Verification items for the finished model (mm, model axes). Face numbers are marked on the shaded views. Round coordinates to 2 decimals unless told otherwise and drop trailing zeros. Order: outer loops, then holes, each group sorted by start corner. A loop starts at its lowest first (then second) coordinate and runs counter-clockwise, first axis right, second up. Notation, with made-up numbers: (59.25, -26) -> (80.25, -26) arc R16 ccw to (80.25, -20) -> close; hole circle Ø6 at (77, 26.5). An arc over 180 degrees is marked (long way). Return JSON: item names as keys, results as strings. Group by question number.
1) Depth check by flat-ended pin: pin 1 (2 mm diameter, centred on x = 5, y = -4, fed in from -Z); pin 2 (5 mm diameter, centred on x = 5, z = -5, fed in from +Y); pin 3 (2 mm diameter, centred on x = 5.5, z = -5.5, fed in from +Y); pin 4 (10 mm diameter, centred on y = 0, z = 0, fed in from -X). Enter the tip coordinate at first touch or a pass-through.
2) Section check A-A on z = 0. Enter the section's corners in (x, y), plus the area to 3 significant figures.
3) Draft check along Y on the marked faces 1, 2 and 3. Enter one of: pulls with the +Y half, pulls with the -Y half, needs draft (parallel to the pull), parting line crosses it, or undercut.
4) Section check B-B on x = 7.25. Enter the section's corners in (y, z), plus the area to 3 significant figures.
5) Section check C-C on x = 5.5. Enter the section's corners in (y, z).
6) Scan lines: L1, parallel to Y at x = 7, z = 0; L2, parallel to Y at x = 3.5, z = 0; L3, parallel to Z at x = 5.25, y = 7. Record each from-to range of solid material in increasing order.
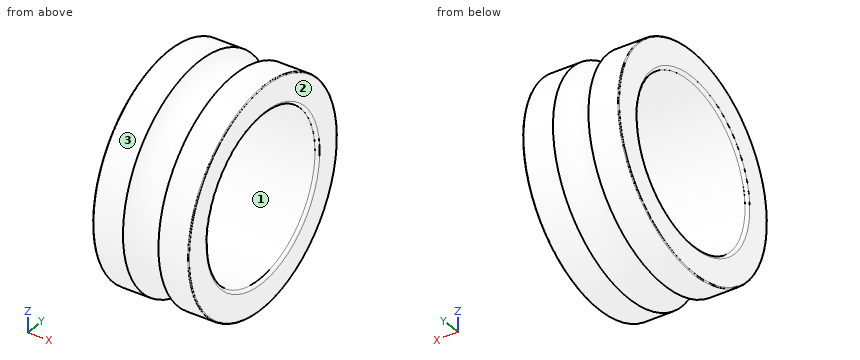
```python
from build123d import *


with BuildPart() as part:
    # Esquisse1 → Révolution1 (revolve)
    with BuildSketch(Plane.XY, mode=Mode.PRIVATE) as r_volution1_sk:
        with BuildLine():
            Line((0.3, 8.5), (9.7, 8.5))
            ThreePointArc((9.7, 8.5), (9.912132034, 8.587867966), (10, 8.8))
            Line((10, 8.8), (10, 11.4))
            ThreePointArc((10, 11.4), (9.970710678, 11.470710678), (9.9, 11.5))
            Line((9.9, 11.5), (6.849097347, 11.5))
            ThreePointArc((6.849097347, 11.5), (5, 10.619), (3.150902653, 11.5))
            Line((3.150902653, 11.5), (0.1, 11.5))
            ThreePointArc((0.1, 11.5), (0.029289322, 11.470710678), (0, 11.4))
            Line((0, 11.4), (0, 8.8))
            ThreePointArc((0, 8.8), (0.087867966, 8.587867966), (0.3, 8.5))
        make_face()
    revolve(r_volution1_sk.sketch.rotate(Axis((100, 0, 0), (-1, 0, 0)), 270), axis=Axis((100, 0, 0), (-1, 0, 0)))


solid = part.part
```
Check result:
{
 "1": {"pin 1": "z = -10.21", "pin 2": "y = 11.01", "pin 3": "y = 9.86", "pin 4": "through"},
 "2": {"outline": "(0, -11.4) arc R0.1 ccw to (0.1, -11.5) -> (3.15, -11.5) arc R2.38 cw to (6.85, -11.5) -> (9.9, -11.5) arc R0.1 ccw to (10, -11.4) -> (10, -8.8) arc R0.3 ccw to (9.7, -8.5) -> (0.3, -8.5) arc R0.3 ccw to (0, -8.8) -> close; (0, 8.8) arc R0.3 ccw to (0.3, 8.5) -> (9.7, 8.5) arc R0.3 ccw to (10, 8.8) -> (10, 11.4) arc R0.1 ccw to (9.9, 11.5) -> (6.85, 11.5) arc R2.38 cw to (3.15, 11.5) -> (0.1, 11.5) arc R0.1 ccw to (0, 11.4) -> close", "area": "55.4 mm^2"},
 "3": {"face 1": "undercut", "face 2": "needs draft", "face 3": "parting line crosses it"},
 "4": {"outline": "circle Ø23 at (0, 0); hole circle Ø17 at (0, 0)", "area": "188 mm^2"},
 "5": {"outline": "circle Ø21.34 at (0, 0); hole circle Ø17 at (0, 0)"},
 "6": {"L1": "-11.5 to -8.5, 8.5 to 11.5", "L2": "-11.15 to -8.5, 8.5 to 11.15", "L3": "-8 to -4.82, 4.82 to 8"}
}
